from build123d import *

# Parameters (mm, degrees)
BOSS_EXTRUDE1_DEPTH = 5.842
SKETCH4_W           = 38.1
SKETCH4_H           = 50.8
SKETCH4_W_2         = 3.048
SKETCH4_H_2         = 76.2
CUT_EXTRUDE2_DEPTH  = 277.973416612


with BuildPart() as part:
    # Sketch3 → Boss-Extrude1 (new body)
    with BuildSketch(Plane.XY):
        with BuildLine():
            Line((0, 241.3), (0, 39.6875))
            Line((0, 39.6875), (135.847173209, 39.6875))
            add(Edge.make_bspline(
                [(0, 241.3), (14.73835438, 241.3), (59.624010151, 216.373546587), (96.769766419, 175.903175742), (127.183964056, 115.738105555), (135.847173209, 66.091328973), (135.847173209, 39.6875)],
                knots=[0, 0, 0, 0, 0.227729534, 0.472592903, 0.661218042, 1, 1, 1, 1], degree=3))
        make_face()
    extrude(amount=BOSS_EXTRUDE1_DEPTH)

    # Sketch4 → Cut-Extrude2 (cut, through all)
    with BuildSketch(Plane.XY):
        with Locations((19.05, 65.0875)):
            Rectangle(SKETCH4_W, SKETCH4_H)
        with Locations((1.524, 203.2)):
            Rectangle(SKETCH4_W_2, SKETCH4_H_2)
    extrude(amount=CUT_EXTRUDE2_DEPTH, mode=Mode.SUBTRACT)

    # Mirror2: part across plane


with BuildPart() as part_1:
    add(part.part)
    add(part.part.mirror(Plane(origin=(0, 0, 0), x_dir=(0, 0, 1), z_dir=(1, 0, 0))))


solid = part_1.part
Design review of the part built by this model. Coordinates are the model's own, in mm. A direction names the side the tool comes from. Round coordinates to 2 decimals unless told otherwise and drop trailing zeros. Return JSON: item names as keys, results as strings. Group by question number.
Item 1: Machinability: for faces 3 (the face through (0, 165.1, 3)), 4 (the face through (1, 90.488, 3)), 5 (the face through (-86, 39.688, 3)), which of the approach directions +Z, -Z, +X, -X, +Y, -Y give a long, thin tool a straight path to every point of the face, cutting with its end or side? Answer none if there is none.
Item 2: Insertion check: P1, Ø3, axis at y = 212.5, z = 2, coming from the -X side; P2, Ø1.5, axis at x = 60.5, z = 4.5, coming from the +Y side; P3, Ø1.8, axis at y = 73, z = 4.5, coming from the -X side. Each pin has a flat end and moves straight along its axis. Give the tip position at first contact, or say it passes through.
Item 3: For probe 1 along X at (y, z) = (87, 3.9); probe 2 along X at (y, z) = (70.5, 2.1); probe 3 along Y at (x, z) = (-86, 4.95), list the stretches that pass through material, from the lowest coordinate up. Write a range as [from, to].
Item 4: The part is to be moulded in two halves that separate along X. For faces 1 (the face through (2, 119, 0)), 2 (the face through (38.1, 65, 3)), say which applies: pulls with the +X half, pulls with the -X half, needs draft (parallel to the pull), parting line crosses it, or undercut.
Model answer:
{
 "1": {"face 3": "+Z, -Z, +Y", "face 4": "+Z, -Z, -Y", "face 5": "+Z, -Z, +X, -X, -Y"},
 "2": {"P1": "stops at x = -60.61", "P2": "stops at y = 211.7", "P3": "stops at x = -133.41"},
 "3": {"probe 1": "x = [-130.84, -38.1], [38.1, 130.84]", "probe 2": "x = [-133.63, -38.1], [38.1, 133.63]", "probe 3": "y = [39.69, 185.88]"},
 "4": {"face 1": "needs draft", "face 2": "undercut"}
}
